```python
from build123d import *

# Parameters (mm, degrees)
F0_W         = 151.6868472099
F0_H         = 67.0943334699
F1_DEPTH     = 25.4
F9_T1_DEPTH  = 212.7476366747
F2_R         = 9.5743665409
F2_R_2       = 9.2989273841
F3_DEPTH     = 25.401
F4_W         = 64.6063834429
F4_H         = 29.3284505606
F10_DEPTH    = 43.7951106578
F11_T1_DEPTH = 140.443628516
F5_R         = 5.2641428602
F6_DEPTH     = 107.9417508016
F8_DEPTH     = 48.2123920152


# Not quite as in the source:
# - a fillet or chamfer that OpenCascade refuses, or shapes differently, is made with other operations: its cross-section is extruded or revolved along the edge and cut away or added


with BuildPart() as f1:
    # F0 (on Top) → F1 (new body)
    with BuildSketch(Plane.XY):
        Rectangle(F0_W, F0_H)
    extrude(amount=F1_DEPTH)

    # F9: fillet of radius 37.4695273349 on 4 edges, made by hand

    # F9_s2 → F9_t1 (cut)
    with BuildSketch(Plane.XY.offset(-93.6738183373)):
        with BuildLine():
            ThreePointArc((75.843423605, -3.9223606), (64.8688531364, 22.5725962664), (38.37389627, 33.5471667349))
            Line((38.37389627, 33.5471667349), (75.843423605, 33.5471667349))
            Line((75.843423605, 33.5471667349), (75.843423605, -3.9223606))
        make_face()
        with BuildLine():
            ThreePointArc((75.843423605, 3.9223606), (64.8688531364, -22.5725962664), (38.37389627, -33.5471667349))
            Line((38.37389627, -33.5471667349), (75.843423605, -33.5471667349))
            Line((75.843423605, -33.5471667349), (75.843423605, 3.9223606))
        make_face()
        with BuildLine():
            ThreePointArc((-75.843423605, 3.9223606), (-64.8688531364, -22.5725962664), (-38.37389627, -33.5471667349))
            Line((-38.37389627, -33.5471667349), (-75.843423605, -33.5471667349))
            Line((-75.843423605, -33.5471667349), (-75.843423605, 3.9223606))
        make_face()
        with BuildLine():
            ThreePointArc((-38.37389627, 33.5471667349), (-64.8688531364, 22.5725962664), (-75.843423605, -3.9223606))
            Line((-75.843423605, -3.9223606), (-75.843423605, 33.5471667349))
            Line((-75.843423605, 33.5471667349), (-38.37389627, 33.5471667349))
        make_face()
    extrude(amount=F9_T1_DEPTH, mode=Mode.SUBTRACT)

    # F2 (on face) → F3 (cut, through all)
    with BuildSketch(Plane.XY.offset(25.4)):
        with Locations((57.8670687973, 0)):
            Circle(F2_R)
        with Locations((-55.8316037059, 0)):
            Circle(F2_R_2)
    extrude(amount=-F3_DEPTH, mode=Mode.SUBTRACT)

    # F4 (on face) → F10 (join)
    with BuildSketch(Plane.XY.offset(25.4)):
        Rectangle(F4_W, F4_H)
    extrude(amount=F10_DEPTH)

    # F11: fillet of radius 15.1674490146 on 2 edges, made by hand

    # F11_s2 → F11_t1 (cut)
    with BuildSketch(Plane.YZ.offset(-70.221814258)):
        with BuildLine():
            ThreePointArc((-14.6642252803, 54.0276616432), (-10.2217823172, 64.7526676947), (0.5032237343, 69.1951106578))
            Line((0.5032237343, 69.1951106578), (-14.6642252803, 69.1951106578))
            Line((-14.6642252803, 69.1951106578), (-14.6642252803, 54.0276616432))
        make_face()
        with BuildLine():
            ThreePointArc((14.6642252803, 54.0276616432), (10.2217823172, 64.7526676947), (-0.5032237343, 69.1951106578))
            Line((-0.5032237343, 69.1951106578), (14.6642252803, 69.1951106578))
            Line((14.6642252803, 69.1951106578), (14.6642252803, 54.0276616432))
        make_face()
    extrude(amount=F11_T1_DEPTH, mode=Mode.SUBTRACT)

    # F5 (on face) → F6 (cut, through all)
    with BuildSketch(Plane.YZ.offset(32.3031917214)):
        with Locations((0, 59.9929094315)):
            Circle(F5_R)
    extrude(amount=-F6_DEPTH, mode=Mode.SUBTRACT)

    # F7 (on face) → F8 (cut, through all)
    with BuildSketch(Plane.XZ.offset(14.6642252803)):
        with BuildLine():
            Line((-10.8441319317, 74.8410969973), (-10.8441319317, 54.0276616432))
            Line((-10.8441319317, 54.0276616432), (-10.6545253, 54.0276616432))
            ThreePointArc((-10.6545253, 54.0276616432), (-1.1741893399, 64.6172881126), (10.3957206011, 56.3617358819))
            Line((10.3957206011, 56.3617358819), (10.3957206011, 74.8410969973))
            Line((10.3957206011, 74.8410969973), (-10.8441319317, 74.8410969973))
        make_face()
        with BuildLine():
            ThreePointArc((10.3957206011, 56.3617358819), (-1.1741893399, 64.6172881126), (-10.6545253, 54.0276616432))
            Line((-10.6545253, 54.0276616432), (10.3957206011, 54.0276616432))
            Line((10.3957206011, 54.0276616432), (10.3957206011, 56.3617358819))
        make_face()
        with BuildLine():
            Line((10.3957206011, 54.0276616432), (-10.6545253, 54.0276616432))
            ThreePointArc((-10.6545253, 54.0276616432), (0, 43.3731363432), (10.6545253, 54.0276616432))
            Line((10.6545253, 54.0276616432), (10.3957206011, 54.0276616432))
        make_face()
    extrude(amount=-F8_DEPTH, mode=Mode.SUBTRACT)


solid = f1.part
```
The listing builds one solid part. Answer for the finished solid, in the listing's coordinates (mm). A direction names the side the tool comes from. Round coordinates to 2 decimals unless told otherwise and drop trailing zeros. Loops run counter-clockwise (first coordinate to the right, second up) from the corner with the lowest first, then second, coordinate; pieces in that order, holes last. Notation, with made-up numbers: (70, 67) -> (101, 67) arc R28 ccw to (101, 104) -> close; hole circle Ø9 at (-11, -21). An arc over 180 degrees is marked (long way). Use one line per item in the form item = value.
1. The part is cut by section A-A on z = 8.5. Determine the outline of the cut face in (x, y), and give its area (3 significant figures).
Answer key:
outline = (-75.64, 0) arc R37.47 ccw to (-38.37, -33.55) -> (38.37, -33.55) arc R37.47 ccw to (75.64, 0) arc R37.47 ccw to (38.37, 33.55) -> (-38.37, 33.55) arc R37.47 ccw to start; hole circle Ø18.6 at (-55.83, 0); hole circle Ø19.15 at (57.87, 0)
area = 8,410 mm²
2. The part is cut by section B-B on y = 7. Determine the outline of the cut face in (x, z), and give its area (3 significant figures).
Answer key:
outline = (-74.22, 0) -> (-61.95, 0) -> (-61.95, 25.4) -> (-74.22, 25.4) -> close; (-49.71, 0) -> (51.33, 0) -> (51.33, 25.4) -> (32.3, 25.4) -> (32.3, 67.21) -> (10.4, 67.21) -> (10.4, 54.03) -> (10.65, 54.03) arc R10.65 cw to (-10.65, 54.03) -> (-10.84, 54.03) -> (-10.84, 67.21) -> (-32.3, 67.21) -> (-32.3, 25.4) -> (-49.71, 25.4) -> close; (64.4, 0) -> (74.22, 0) -> (74.22, 25.4) -> (64.4, 25.4) -> close
area = 5,370 mm²
3. The part is cut by section D-D on x = -56.5. Determine the outline of the cut face in (y, z), and give its area (3 significant figures).
Answer key:
outline = (-28.87, 0) -> (-9.27, 0) -> (-9.27, 25.4) -> (-28.87, 25.4) -> close; (9.27, 0) -> (28.87, 0) -> (28.87, 25.4) -> (9.27, 25.4) -> close
area = 995 mm²
4. Flat-ended cylindrical pins translate along their axes: pin 1 Ø12 at (y, z) = (6, 63) entering from -X; pin 2 Ø1.5 at (y, z) = (8.5, 56) entering from +X; pin 3 Ø3 at (x, y) = (26.5, 11) entering from +Z; pin 4 Ø8.5 at (y, z) = (0, 59.99) entering from -X. Find the tip coordinate at first contact, or state that the pin passes through.
Answer key:
pin_1 = -32.3
pin_2 = 32.3
pin_3 = 65.43
pin_4 = through
5. The part is cut by section C-C on x = -14.5. Determine the outline of the cut face in (y, z).
Answer key:
outline = (-33.55, 0) -> (33.55, 0) -> (33.55, 25.4) -> (14.66, 25.4) -> (14.66, 54.03) arc R15.17 ccw to (0, 69.19) arc R15.17 ccw to (-14.66, 54.03) -> (-14.66, 25.4) -> (-33.55, 25.4) -> close; hole circle Ø10.53 at (0, 59.99)
6. Find the intervals of material crossed by probe 1 along Z at (x, y) = (47.5, 7); probe 2 along Y at (x, z) = (12, 48.5); probe 3 along X at (y, z) = (-11, 63.5), in increasing order. Write a range as [from, to].
Answer key:
probe_1 = [0, 25.4]
probe_2 = [-14.66, 14.66]
probe_3 = [-32.3, -10.84], [10.4, 32.3]
7. A tool of negligible diameter and unlimited length cuts with its end or side. For faces 4 (the flat face through (0, -14.664, 40)), 5 (the flat face through (32.303, 0, 42)), 6 (the flat face through (10.396, -3, 65)), 7 (the flat face through (-32.303, 0, 42)), from which of +Z, -Z, +X, -X, +Y, -Y can it reach the whole face along a straight path? Write none if from no direction.
Answer key:
face_4 = +Z, +X, -X, -Y
face_5 = +Z, +X, +Y, -Y
face_6 = +Z, +Y, -Y
face_7 = +Z, -X, +Y, -Y
8. For a pull along X with two mould halves and no side action, classify faces 1 (the cylindrical face through (63.728, 23.666, 12.522)), 2 (the cylindrical face through (-21.724, -10.511, 64.455)), 3 (the cylindrical face through (67, 2.88, 12.88)) as released by +X, released by -X, zero draft, split by the parting line, or undercut.
Answer key:
face_1 = released by +X
face_2 = zero draft
face_3 = undercut
